Autodesk Inventor part; units mm, degrees
ref_plane "YZ Plane" through (0, 0, 0) normal (1, 0, 0) x (0, 1, 0)
ref_plane "XZ Plane" through (0, 0, 0) normal (0, 1, 0) x (-1, 0, 0)
ref_plane "XY Plane" through (0, 0, 0) normal (0, 0, 1) x (1, 0, 0)
sketch "Sketch1" plane through (0, 0, 0) normal (0, 1, 0) x (-1, 0, 0)
  line L0 (0, 52.8555) -> (50.8, 52.8555)
  line L1 (50.8, 52.8555) -> (50.8, -74.1445)
  line L2 (50.8, -74.1445) -> (0, -74.1445)
  line L3 (0, -74.1445) -> (0, 52.8555)
  point P0 (0, 0)
  dimension "d0" = 50.8
  dimension "d1" = 127
extrude "Extrusion1" add sketch "Sketch1" along normal blind 6.35
sketch "Sketch2" plane through (0, 6.35, 0) normal (0, 1, 0) x (1, 0, 0)
  line L0 (-50.8, -52.8555) -> (0, -52.8555)
  line L1 (0, 74.1445) -> (-50.8, 74.1445)
  line L2 (0, -52.8555) -> (-10.16, -52.8555)
  line L3 (-10.16, -52.8555) -> (-10.16, 74.1445)
  line L4 (-10.16, 74.1445) -> (0, 74.1445)
  line L5 (0, 74.1445) -> (0, -52.8555)
  line L6 (-50.8, 74.1445) -> (-40.64, 74.1445)
  line L7 (-40.64, 74.1445) -> (-40.64, -52.8555)
  line L8 (-40.64, -52.8555) -> (-50.8, -52.8555)
  line L9 (-50.8, -52.8555) -> (-50.8, 74.1445)
  point P0 (0, 0)
  point P1 (-40.64, -52.8555)
  dimension "d4" = 10.16
  dimension "d5" = 10.16
extrude "Extrusion2" add sketch "Sketch2" along normal blind 25.4 contours L9 L1 L7 L0 | L3 L1 L5 L0
sketch "Sketch3" plane through (-40.64, 6.35, 52.8555) normal (1, 0, 0) x (0, 0, -1)
  line L0 (127, 25.4) -> (0, 25.4)
  line L1 (0, 25.4) -> (127, 25.4)
  line L2 (127, 25.4) -> (127, 19.05)
  line L3 (127, 19.05) -> (0, 19.05)
  line L4 (0, 19.05) -> (0, 25.4)
  point P0 (52.8555, -6.35)
  dimension "d8" = 6.35
extrude "Extrusion3" add sketch "Sketch3" along normal blind 6.35
sketch "Sketch4" plane through (-10.16, 6.35, -74.1445) normal (-1, 0, 0) x (0, 0, 1)
  line L0 (0, 25.4) -> (127, 25.4)
  line L1 (127, 25.4) -> (127, 19.05)
  line L2 (0, 25.4) -> (127, 25.4)
  line L3 (127, 25.4) -> (127, 19.05)
  line L4 (127, 19.05) -> (0, 19.05)
  line L5 (0, 19.05) -> (0, 25.4)
  point P0 (74.1445, -6.35)
extrude "Extrusion4" add sketch "Sketch4" along normal blind 6.35
sketch "Sketch5" plane through (0, 0, 0) normal (0, -1, 0) x (1, 0, 0)
  circle A0 centre (-25.4, -10.6445) radius 8.729
  line L0 (0, 52.8555) -> (0, -74.1445)
  line L1 (0, -74.1445) -> (-50.8, -74.1445)
  point P0 (0, 0)
  dimension "d13" = 25.4
  dimension "d14" = 63.5
extrude "Extrusion5" cut sketch "Sketch5" against normal up to surface (6.35 mm away)
properties part number "jeep pvc connector"
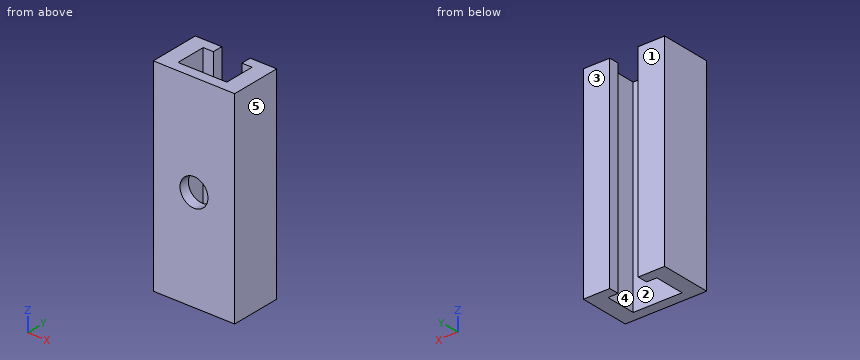
Model file for the job. Use its own axes, mm. Face numbers are marked on the shaded views. A direction names the side the tool comes from. Coordinates: 2 decimals unless noted, no trailing zeros. Write each loop counter-clockwise with the first axis right and the second up, starting at its lowest first coordinate (ties: lowest second). Pieces come first, ordered by that corner, then holes. Notation, with made-up numbers: (-2.5, 45) - (29.5, 45) arc R11 cw to (29.5, 62) - close; hole circle Ø2 at (71, 31.25). An arc over 180 degrees is marked (long way). One line per question, with ' | ' between items. Start each with the question number.
Q1. Cut at B-B, the plane y = 28. List the corners of the cut face in (x, z).
Q2. Cut at C-C, the plane z = 1. List the corners of the cut face in (x, y).
Q3. Drill centre lines: line 1 (X direction, y = 28, z = 5); line 2 (Y direction, x = -13.5, z = -55); line 3 (X direction, y = 18, z = -22). Where is each one in solid material? Low to high. Write a range as [from, to].
Q4. Cut at A-A, the plane x = -25.4. List the corners of the cut face in (y, z).
Q5. 3-axis set-ups, long thin cutter, end or side, ignore diameter. For the marked faces 1 and 2: which of +Z, -Z, +X, -X, +Y, -Y reach the whole face in a straight line?
Q6. Pull direction X, two halves, no side cores. Call the marked faces 3, 4 and 5: pulls with the +X half, pulls with the -X half, needs draft (parallel to the pull), parting line crosses it, or undercut.
Answer below:
1) outline: (-50.8, -74.14) - (-34.29, -74.14) - (-34.29, 52.86) - (-50.8, 52.86) - close; (-16.51, -74.14) - (0, -74.14) - (0, 52.86) - (-16.51, 52.86) - close
2) outline: (-50.8, 0) - (0, 0) - (0, 31.75) - (-16.51, 31.75) - (-16.51, 25.4) - (-10.16, 25.4) - (-10.16, 6.35) - (-40.64, 6.35) - (-40.64, 25.4) - (-34.29, 25.4) - (-34.29, 31.75) - (-50.8, 31.75) - close
3) line 1: [-50.8, -34.29], [-16.51, 0] | line 2: [0, 6.35], [25.4, 31.75] | line 3: [-50.8, -40.64], [-10.16, 0]
4) outline: (0, -74.14) - (6.35, -74.14) - (6.35, -19.37) - (0, -19.37) - close; (0, -1.92) - (6.35, -1.92) - (6.35, 52.86) - (0, 52.86) - close
5) face 1: +Z, -Z, +X, -X, +Y | face 2: +Z, -Z
6) face 3: needs draft | face 4: undercut | face 5: pulls with the +X half
